from build123d import *

# Parameters (mm, degrees)
SKETCH_1_R               = 7.9
EXTRUDE_1_DEPTH          = 20
SKETCH_3_R               = 10
EXTRUDE_2_DEPTH          = 2
EXTRUDE_3_DEPTH          = 15
CHAMFER_1_SIZE           = 0.5
M5X0_8_1_D               = 4.2
M5X0_8_1_DEPTH           = 12.4
M5X0_8_1_TIP             = 1.2618073
SKETCH_5_R               = 3.1
CUT_EXTRUDE_1_DEPTH      = 11
CUT_EXTRUDE_1_DEPTH_BACK = 11
CHAMFER_2_SIZE           = 1


with BuildPart() as part:
    # 草图1 → 凸台-拉伸1 (new body)
    with BuildSketch(Plane(origin=(0, 0, 0), x_dir=(0, 0, -1), z_dir=(1, 0, 0))):
        Circle(SKETCH_1_R)
    extrude(amount=EXTRUDE_1_DEPTH)

    # 草图3 → 凸台-拉伸2 (add)
    with BuildSketch(Plane.ZY):
        Circle(SKETCH_3_R)
    extrude(amount=EXTRUDE_2_DEPTH)

    # 草图4 → 凸台-拉伸3 (add)
    with BuildSketch(Plane.ZY.offset(2)):
        Polygon((6.35, 3.666174209), (0, 7.332348419), (-6.35, 3.666174209), (-6.35, -3.666174209), (0, -7.332348419), (6.35, -3.666174209), align=None)
    extrude(amount=EXTRUDE_3_DEPTH)

    # 倒角1
    chamfer_1_edges = [part.edges().sort_by_distance(p)[0] for p in [
        (-2, 0, -10),
    ]]
    chamfer(chamfer_1_edges, length=CHAMFER_1_SIZE)

    # M5x0.8 螺纹孔1
    with Locations(Plane.ZY.offset(17)):
        with Locations((0, 0)):
            Hole(M5X0_8_1_D / 2, depth=M5X0_8_1_DEPTH)
            with Locations((0, 0, -(M5X0_8_1_DEPTH + M5X0_8_1_TIP / 2))):  # 118° drill point
                Cone(0, M5X0_8_1_D / 2, M5X0_8_1_TIP, mode=Mode.SUBTRACT)

    # 草图5 → 切除-拉伸1 (cut, two sides)
    with BuildSketch(Plane(origin=(0, 0, 0), x_dir=(1, 0, 0), z_dir=(0, 1, 0))) as cut_extrude_1_sk:
        with Locations((10, 0)):
            Circle(SKETCH_5_R)
    extrude(amount=CUT_EXTRUDE_1_DEPTH, mode=Mode.SUBTRACT)
    extrude(cut_extrude_1_sk.sketch, amount=-CUT_EXTRUDE_1_DEPTH_BACK, mode=Mode.SUBTRACT)

    # 倒角2
    chamfer_2_edges = [part.edges().sort_by_distance(p)[0] for p in [
        (20, 0, 7.9),
    ]]
    chamfer(chamfer_2_edges, length=CHAMFER_2_SIZE)


solid = part.part
Design review of the part built by this model. Coordinates are the model's own, in mm. A direction names the side the tool comes from. Round coordinates to 2 decimals unless told otherwise and drop trailing zeros. Order: outer loops, then holes, each group sorted by start corner. A loop starts at its lowest first (then second) coordinate and runs counter-clockwise, first axis right, second up. Notation, with made-up numbers: M 13,64.25 L 37,64.25 A31 cw 37,88.25 Z; hole C 8,15.5 d3. An arc over 180 degrees is marked long. Answer as CSV lines item,"result". Start each with the question number.
1) For pin 1 Ø7 at (x, z) = (10, 0) entering from -Y; pin 2 Ø3 at (x, y) = (-6.5, 1) entering from -Z; pin 3 Ø6 at (x, z) = (-12, -5) entering from -Y, all flat-tipped, find the tip position at first contact; note any pin that passes through.
2) Add section A-A (x = -11.5). Give the boundary of the cut face in (y, z).
3) Add section B-B (x = 4). Give the boundary of the cut face in (y, z), then the cut area to 3 significant figures.
4) Add section C-C (x = 10). Give the boundary of the cut face in (y, z).
5) The part is to be moulded in two halves that separate along Y. For faces 1 (the face through (-17, -2, -2)), 2 (the face through (-3.56, 0.11, 0.35)), 3 (the face through (9.367, -7.009, -3.645)), 4 (the face through (-9.395, 5.474, 3.219)), say which applies: +Y half, -Y half, draft (parallel to the pull), parting line (faces both ways), or undercut.
6) Tool access review of faces 5 (the face through (0, -4, 7)), 6 (the face through (-9, 0, 6.35)), 7 (the face through (-9.395, 5.525, -3.131)): name each direction out of +Z, -Z, +X, -X, +Y, -Y from which nothing blocks a thin tool from reaching the whole face with its end or side.
7) Wall thickness on line 1 along Z through (x, y) = (-14.25, 0); line 2 along Y through (x, z) = (-7.5, 0); line 3 along X through (y, z) = (3.25, 0.5): over which ranges is each line inside the solid? List them lowest first. Write a range as [from, to].
Resolved:
1,pin 1,"y = -7.9"
1,pin 2,"z = -6.35"
1,pin 3,"y = -6.18"
2,outline,"M -7.33,0 L -3.67,-6.35 L 3.67,-6.35 L 7.33,0 L 3.67,6.35 L -3.67,6.35 Z; hole C 0,0 d4.2"
3,outline,"C 0,0 d15.8"
3,area,"196 mm^2"
4,outline,"M -7.27,-3.1 A7.9 ccw 7.27,-3.1 Z; M -7.27,3.1 L 7.27,3.1 A7.9 ccw Z"
5,face 1,"draft"
5,face 2,"undercut"
5,face 3,"parting line"
5,face 4,"+Y half"
6,face 5,"+X"
6,face 6,"+Z, -X, +Y, -Y"
6,face 7,"-Z, -X, +Y"
7,line 1,"[-6.35, -2.1], [2.1, 6.35]"
7,line 2,"[-7.33, -2.1], [2.1, 7.33]"
7,line 3,"[-17, 6.94], [13.06, 20]"
